```python
from build123d import *

# Parameters (mm, degrees)
F1_DEPTH = 8
F2_R     = 9.5
F2_R_2   = 3.2
F3_DEPTH = 8
F4_W     = 0.682370679
F4_H     = 6.463566795
F5_DEPTH = 2


with BuildPart() as f1:
    # F0 (on Top) → F1 (new body)
    with BuildSketch(Plane.XY):
        with BuildLine():
            ThreePointArc((20.6296333293, -0.9169125905), (20.6449077044, -0.4585693786), (20.65, 0))
            ThreePointArc((20.65, 0), (20.0407277838, 4.9791294317), (18.2488639325, 9.6644433453))
            ThreePointArc((18.2488639325, 9.6644433453), (16.899563072, 10.0263287386), (17.228671645, 11.3839963699))
            ThreePointArc((17.228671645, 11.3839963699), (13.6343948602, 15.5088934743), (9.0830237721, 18.5451120017))
            ThreePointArc((9.0830237721, 18.5451120017), (7.7787055485, 18.0447842877), (7.2469429653, 19.3366056395))
            ThreePointArc((7.2469429653, 19.3366056395), (1.9145582783, 20.5610546081), (-3.5522227527, 20.34217819))
            ThreePointArc((-3.5522227527, 20.34217819), (-3.537714089, 20.2447444729), (-3.5328621738, 20.1463560108))
            ThreePointArc((-3.5328621738, 20.1463560108), (-4.4104069619, 19.1538819703), (-5.5028716159, 19.9032887729))
            ThreePointArc((-5.5028716159, 19.9032887729), (-10.5365744934, 17.7595917167), (-14.83064092, 14.3692237056))
            ThreePointArc((-14.83064092, 14.3692237056), (-14.5928551239, 14.0354855032), (-14.5088934877, 13.634394845))
            ThreePointArc((-14.5088934877, 13.634394845), (-15.0857403153, 12.7283366831), (-16.1507762731, 12.8675920738))
            ThreePointArc((-16.1507762731, 12.8675920738), (-18.9630939126, 8.1745684449), (-20.4442583125, 2.9077142313))
            ThreePointArc((-20.4442583125, 2.9077142313), (-19.813794176, 2.5790896437), (-19.5610546025, 1.9145583389))
            ThreePointArc((-19.5610546025, 1.9145583389), (-19.8786246519, 1.1836073402), (-20.6296333275, 0.916912631))
            ThreePointArc((-20.6296333275, 0.916912631), (-20.1463560242, -4.5328621144), (-18.2488639515, -9.6644433094))
            ThreePointArc((-18.2488639515, -9.6644433094), (-17.2542563165, -9.6736514422), (-16.7595917478, -10.536574441))
            ThreePointArc((-16.7595917478, -10.536574441), (-16.8846860156, -11.020867699), (-17.2286716673, -11.383996336))
            ThreePointArc((-17.2286716673, -11.383996336), (-13.6343948907, -15.5088934475), (-9.0830238086, -18.5451119838))
            ThreePointArc((-9.0830238086, -18.5451119838), (-7.9606237803, -17.9862481273), (-7.1745684636, -18.9630939046))
            ThreePointArc((-7.1745684636, -18.9630939046), (-7.1928288188, -19.1533234235), (-7.2469430033, -19.3366056253))
            ThreePointArc((-7.2469430033, -19.3366056253), (-1.9145583187, -20.5610546044), (3.5522227127, -20.342178197))
            ThreePointArc((3.5522227127, -20.342178197), (4.313353072, -19.1707455587), (5.5028715768, -19.9032887837))
            ThreePointArc((5.5028715768, -19.9032887837), (10.5365744585, -17.7595917375), (14.8306408918, -14.3692237348))
            ThreePointArc((14.8306408918, -14.3692237348), (14.7578574579, -12.9741336224), (16.1507762478, -12.8675921056))
            ThreePointArc((16.1507762478, -12.8675921056), (18.9630939126, -8.1745684449), (20.4442583182, -2.9077141911))
            ThreePointArc((20.4442583182, -2.9077141911), (19.5653618893, -1.8218436109), (20.6296333293, -0.9169125905))
        make_face()
        with BuildLine():
            ThreePointArc((17.228671645, 11.3839963699), (16.899563072, 10.0263287386), (18.2488639325, 9.6644433453))
            ThreePointArc((18.2488639325, 9.6644433453), (17.7595917271, 10.5365744759), (17.228671645, 11.3839963699))
        make_face()
        with BuildLine():
            ThreePointArc((17.228671645, 11.3839963699), (17.7595917271, 10.5365744759), (18.2488639325, 9.6644433453))
            ThreePointArc((18.2488639325, 9.6644433453), (18.6225147264, 10.0312390454), (18.7595917271, 10.5365744759))
            ThreePointArc((18.7595917271, 10.5365744759), (18.2438849843, 11.4114802086), (17.228671645, 11.3839963699))
        make_face()
        with BuildLine():
            ThreePointArc((21.5610546063, -1.9145582985), (21.2920056043, -1.2321283472), (20.6296333293, -0.9169125905))
            ThreePointArc((20.6296333293, -0.9169125905), (20.5610546063, -1.9145582985), (20.4442583182, -2.9077141911))
            ThreePointArc((20.4442583182, -2.9077141911), (21.2255859118, -2.6618187243), (21.5610546063, -1.9145582985))
        make_face()
        with BuildLine():
            ThreePointArc((20.4442583182, -2.9077141911), (20.5610546063, -1.9145582985), (20.6296333293, -0.9169125905))
            ThreePointArc((20.6296333293, -0.9169125905), (19.5653618893, -1.8218436109), (20.4442583182, -2.9077141911))
        make_face()
        with BuildLine():
            ThreePointArc((7.2469429653, 19.3366056395), (7.7787055485, 18.0447842877), (9.0830237721, 18.5451120017))
            ThreePointArc((9.0830237721, 18.5451120017), (8.1745684263, 18.9630939207), (7.2469429653, 19.3366056395))
        make_face()
        with BuildLine():
            ThreePointArc((7.2469429653, 19.3366056395), (8.1745684263, 18.9630939207), (9.0830237721, 18.5451120017))
            ThreePointArc((9.0830237721, 18.5451120017), (9.1514142038, 18.7491492384), (9.1745684263, 18.9630939207))
            ThreePointArc((9.1745684263, 18.9630939207), (8.3647979443, 19.9448335656), (7.2469429653, 19.3366056395))
        make_face()
        with BuildLine():
            ThreePointArc((16.5088934609, -13.6343948754), (16.4149516232, -13.2112417039), (16.1507762478, -12.8675921056))
            ThreePointArc((16.1507762478, -12.8675921056), (15.5088934609, -13.6343948754), (14.8306408918, -14.3692237348))
            ThreePointArc((14.8306408918, -14.3692237348), (15.9099841183, -14.5504332396), (16.5088934609, -13.6343948754))
        make_face()
        with BuildLine():
            ThreePointArc((14.8306408918, -14.3692237348), (15.5088934609, -13.6343948754), (16.1507762478, -12.8675921056))
            ThreePointArc((16.1507762478, -12.8675921056), (14.7578574579, -12.9741336224), (14.8306408918, -14.3692237348))
        make_face()
        with BuildLine():
            ThreePointArc((-3.5328621738, 20.1463560108), (-3.537714089, 20.2447444729), (-3.5522227527, 20.34217819))
            ThreePointArc((-3.5522227527, 20.34217819), (-4.5328621738, 20.1463560108), (-5.5028716159, 19.9032887729))
            ThreePointArc((-5.5028716159, 19.9032887729), (-4.4104069619, 19.1538819703), (-3.5328621738, 20.1463560108))
        make_face()
        with BuildLine():
            ThreePointArc((-5.5028716159, 19.9032887729), (-4.5328621738, 20.1463560108), (-3.5522227527, 20.34217819))
            ThreePointArc((-3.5522227527, 20.34217819), (-4.7523712379, 21.1219664714), (-5.5028716159, 19.9032887729))
        make_face()
        with BuildLine():
            ThreePointArc((5.5328621342, -20.1463560197), (5.5253361748, -20.0239008088), (5.5028715768, -19.9032887837))
            ThreePointArc((5.5028715768, -19.9032887837), (4.5328621342, -20.1463560197), (3.5522227127, -20.342178197))
            ThreePointArc((3.5522227127, -20.342178197), (4.6312505953, -21.1415041045), (5.5328621342, -20.1463560197))
        make_face()
        with BuildLine():
            ThreePointArc((3.5522227127, -20.342178197), (4.5328621342, -20.1463560197), (5.5028715768, -19.9032887837))
            ThreePointArc((5.5028715768, -19.9032887837), (4.313353072, -19.1707455587), (3.5522227127, -20.342178197))
        make_face()
        with BuildLine():
            ThreePointArc((-14.5088934877, 13.634394845), (-14.5928551239, 14.0354855032), (-14.83064092, 14.3692237056))
            ThreePointArc((-14.83064092, 14.3692237056), (-15.5088934877, 13.634394845), (-16.1507762731, 12.8675920738))
            ThreePointArc((-16.1507762731, 12.8675920738), (-15.0857403153, 12.7283366831), (-14.5088934877, 13.634394845))
        make_face()
        with BuildLine():
            ThreePointArc((-16.1507762731, 12.8675920738), (-15.5088934877, 13.634394845), (-14.83064092, 14.3692237056))
            ThreePointArc((-14.83064092, 14.3692237056), (-16.2599294919, 14.2946560965), (-16.1507762731, 12.8675920738))
        make_face()
        with BuildLine():
            ThreePointArc((-9.0830238086, -18.5451119838), (-8.5704313432, -19.8814035368), (-7.2469430033, -19.3366056253))
            ThreePointArc((-7.2469430033, -19.3366056253), (-8.1745684636, -18.9630939046), (-9.0830238086, -18.5451119838))
        make_face()
        with BuildLine():
            ThreePointArc((-9.0830238086, -18.5451119838), (-8.1745684636, -18.9630939046), (-7.2469430033, -19.3366056253))
            ThreePointArc((-7.2469430033, -19.3366056253), (-7.1928288188, -19.1533234235), (-7.1745684636, -18.9630939046))
            ThreePointArc((-7.1745684636, -18.9630939046), (-7.9606237803, -17.9862481273), (-9.0830238086, -18.5451119838))
        make_face()
        with BuildLine():
            ThreePointArc((-19.5610546025, 1.9145583389), (-19.813794176, 2.5790896437), (-20.4442583125, 2.9077142313))
            ThreePointArc((-20.4442583125, 2.9077142313), (-20.5610546025, 1.9145583389), (-20.6296333275, 0.916912631))
            ThreePointArc((-20.6296333275, 0.916912631), (-19.8786246519, 1.1836073402), (-19.5610546025, 1.9145583389))
        make_face()
        with BuildLine():
            ThreePointArc((-20.6296333275, 0.916912631), (-20.5610546025, 1.9145583389), (-20.4442583125, 2.9077142313))
            ThreePointArc((-20.4442583125, 2.9077142313), (-21.5567473193, 2.0072730284), (-20.6296333275, 0.916912631))
        make_face()
        with BuildLine():
            ThreePointArc((-18.2488639515, -9.6644433094), (-18.6196204039, -11.0468201767), (-17.2286716673, -11.383996336))
            ThreePointArc((-17.2286716673, -11.383996336), (-17.7595917478, -10.536574441), (-18.2488639515, -9.6644433094))
        make_face()
        with BuildLine():
            ThreePointArc((-18.2488639515, -9.6644433094), (-17.7595917478, -10.536574441), (-17.2286716673, -11.383996336))
            ThreePointArc((-17.2286716673, -11.383996336), (-16.8846860156, -11.020867699), (-16.7595917478, -10.536574441))
            ThreePointArc((-16.7595917478, -10.536574441), (-17.2542563165, -9.6736514422), (-18.2488639515, -9.6644433094))
        make_face()
    extrude(amount=F1_DEPTH)

    # F2 (on face) → F3 (join)
    with BuildSketch(Plane.XY.offset(8)):
        Circle(F2_R)
        Circle(F2_R_2, mode=Mode.SUBTRACT)
    extrude(amount=F3_DEPTH)

    # F4 (on face) → F5 (join)
    with BuildSketch(Plane.XY.offset(8)):
        with Locations((-0.0285869173, -0.0104163773)):
            Rectangle(F4_W, F4_H)
    extrude(amount=F5_DEPTH)


solid = f1.part
```
Geometry check sheet. Reference: the model listing, model coordinates, mm. A direction names the side the tool comes from. Give positions to 0.01 mm unless a question says otherwise; leave off trailing zeros. Loops run counter-clockwise (first coordinate to the right, second up) from the corner with the lowest first, then second, coordinate; pieces in that order, holes last. Notation, with made-up numbers: M 65.5,73.5 L 83.5,73.5 A25 cw 83.5,105.5 Z; hole C -10,31.5 d9. An arc over 180 degrees is marked long. Write item = value, one per line. Start each with the question number.
1. Section check A-A, the plane z = 9.5. Enter the section's corners in (x, y), plus the area to 3 significant figures.
2. Go/stop test with flat-tipped pins: P1, Ø5, axis at x = 15, z = 3.5, coming from the -Y side; P2, Ø0.6, axis at y = -1, z = 9.5, coming from the +X side; P3, Ø0.6, axis at y = 0.5, z = 9, coming from the -X side. Record where each tip stops, or that it passes through.
3. Tool access check on faces 1 (the face through (-20.163, -4.458, 3.944)), 2 (the face through (0, 10, 8)), 3 (the face through (-16.245, 14.311, 3.944)). Record the directions out of +Z, -Z, +X, -X, +Y, -Y that give a thin tool (end or side, any length) a straight path to the whole face; none if there is none.
4. Thickness scan on probe 1 along Y at (x, z) = (0, 11.75); probe 2 along Z at (x, y) = (1.5, -0.5); probe 3 along Y at (x, z) = (1.5, 9.5). Record the ranges inside material, lowest first.
5. Section check C-C, the plane z = 6.5. Enter the section's corners in (x, y), plus the area to 3 significant figures.
6. Section check B-B, the plane y = 9. Enter the section's corners in (x, z).
7. Section check D-D, the plane x = -5. Enter the section's corners in (y, z).
8. Draft check along Y on faces 4 (the face through (1.991, 20.554, 3.944)), 5 (the face through (-1, 0, 8)), 6 (the face through (4, 0, 16)), 7 (the face through (-18.63, -11.03, 3.94)). Enter one of: +Y half, -Y half, draft (parallel to the pull), parting line (faces both ways), or undercut.
Values follow:
q1.outline = C 0,0 d19; hole M -0.37,-3.18 L -0.37,3.18 A3.2 ccw Z; hole M 0.31,-3.18 A3.2 ccw 0.31,3.18 Z
q1.area = 256 mm^2
q2.P1 = -16.44
q2.P2 = 9.47
q2.P3 = -9.5
q3.face_1 = +Z, -Z, -X
q3.face_2 = +Z
q3.face_3 = +Z, -Z
q4.probe_1 = -9.5 to -3.2, 3.2 to 9.5
q4.probe_2 = 0 to 8
q4.probe_3 = -9.38 to -2.83, 2.83 to 9.38
q5.outline = M -20.63,0.92 A20.65 ccw -18.25,-9.66 A1 ccw long -17.23,-11.38 A20.65 ccw -9.08,-18.55 A1 ccw long -7.25,-19.34 A20.65 ccw 3.55,-20.34 A1 ccw long 5.5,-19.9 A20.65 ccw 14.83,-14.37 A1 ccw long 16.15,-12.87 A20.65 ccw 20.44,-2.91 A1 ccw long 20.63,-0.92 A20.65 ccw 18.25,9.66 A1 ccw long 17.23,11.38 A20.65 ccw 9.08,18.55 A1 ccw long 7.25,19.34 A20.65 ccw -3.55,20.34 A1 ccw long -5.5,19.9 A20.65 ccw -14.83,14.37 A1 ccw long -16.15,12.87 A20.65 ccw -20.44,2.91 A1 ccw long Z
q5.area = 1,360 mm^2
q6.outline = M -18.59,0 L 18.59,0 L 18.59,8 L 3.04,8 L 3.04,16 L -3.04,16 L -3.04,8 L -18.59,8 Z
q7.outline = M -20.04,0 L 21.03,0 L 21.03,8 L 8.08,8 L 8.08,16 L -8.08,16 L -8.08,8 L -20.04,8 Z
q8.face_4 = +Y half
q8.face_5 = undercut
q8.face_6 = draft
q8.face_7 = undercut
